```python
from build123d import *

# Parameters (mm, degrees)
F1_DEPTH = 20
F2_R     = 3


with BuildPart() as f1:
    # F0 (on Front) → F1 (new body)
    with BuildSketch(Plane.XZ):
        with BuildLine():
            Line((0, 50), (0, 0))
            Line((0, 0), (200, 0))
            Line((200, 0), (200, 17.131216))
            ThreePointArc((200, 17.131216), (196.384482, 26.898179), (187.280858, 31.956791))
            Line((187.280858, 31.956791), (82.719142, 48.043209))
            ThreePointArc((82.719142, 48.043209), (73.615518, 53.101821), (70, 62.868784))
            Line((70, 62.868784), (70, 137.131216))
            ThreePointArc((70, 137.131216), (73.615518, 146.898179), (82.719142, 151.956791))
            Line((82.719142, 151.956791), (187.280858, 168.043209))
            ThreePointArc((187.280858, 168.043209), (196.384482, 173.101821), (200, 182.868784))
            Line((200, 182.868784), (200, 200))
            Line((200, 200), (0, 200))
            Line((0, 200), (0, 150))
            Line((0, 150), (20, 150))
            Line((20, 150), (20, 50))
            Line((20, 50), (0, 50))
        make_face()
    extrude(amount=F1_DEPTH)

    # F2
    f2_edges = [f1.edges().sort_by_distance(p)[0] for p in [
        (196.384482, -20, 173.101821),
        (200, -20, 191.434392),
        (100, -20, 200),
        (0, -20, 175),
        (10, -20, 150),
        (20, -20, 100),
        (10, -20, 50),
        (0, -20, 25),
        (100, -20, 0),
        (200, -20, 8.565608),
        (196.384482, -20, 26.898179),
        (135, -20, 40),
        (73.615518, -20, 53.101821),
        (70, -20, 100),
        (73.615518, -20, 146.898179),
        (135, -20, 160),
        (196.384482, 0, 173.101821),
        (200, 0, 191.434392),
        (100, 0, 200),
        (0, 0, 175),
        (10, 0, 150),
        (20, 0, 100),
        (10, 0, 50),
        (0, 0, 25),
        (100, 0, 0),
        (200, 0, 8.565608),
        (196.384482, 0, 26.898179),
        (135, 0, 40),
        (73.615518, 0, 53.101821),
        (70, 0, 100),
        (73.615518, 0, 146.898179),
        (135, 0, 160),
    ]]
    fillet(f2_edges, radius=F2_R)


solid = f1.part
```
Check sheet for the modelled part. Datum: model origin and axes. Units: mm. A direction names the side the tool comes from. Round coordinates to 2 decimals unless told otherwise and drop trailing zeros. Order: outer loops, then holes, each group sorted by start corner. A loop starts at its lowest first (then second) coordinate and runs counter-clockwise, first axis right, second up.
1) Section check B-B (z = 74). Record the boundary of the cut face in (x, y), and give its area (3 significant figures).
2) Scan lines: line 1 (Z direction, x = 139.5, y = -4.25); line 2 (Z direction, x = 185.5, y = -16.5); line 3 (X direction, y = -8.75, z = 70.5). Record each from-to range of solid material in increasing order.
3) Mould release check, pull along Z, two halves, no side actions. Record for faces 4 (the cylindrical face through (196.29, -9.9, 172.99)), 5 (the flat face through (200, -10, 8)), 6 (the flat face through (99, -10, 0)), 7 (the cylindrical face through (135.6, -19.1, 160.96)): +Z half, -Z half, draft (parallel to the pull), parting line (faces both ways), or undercut.
4) Section check A-A (y = -10.5). Record the boundary of the cut face in (x, z), and give its area (3 significant figures).
5) Go/stop test with flat-tipped pins: pin 1 Ø8 at (x, y) = (128, -2.5) entering from -Z; pin 2 Ø4 at (y, z) = (-12, 88.5) entering from -X; pin 3 Ø5 at (y, z) = (-3.5, 100.5) entering from +X. Record where each tip stops, or that it passes through.
6) Tool access check on faces 1 (the flat face through (20, -10, 101)), 2 (the cylindrical face through (134.138, -0.902, 39.267)), 3 (the cylindrical face through (73.519, -9.902, 146.785)). Record the directions out of +Z, -Z, +X, -X, +Y, -Y that give a thin tool (end or side, any length) a straight path to the whole face; none if there is none.
Result:
1. outline: (20, -17) arc R3 ccw to (23, -20) - (67, -20) arc R3 ccw to (70, -17) - (70, -3) arc R3 ccw to (67, 0) - (23, 0) arc R3 ccw to (20, -3) - close
1. area: 992 mm2
2. line 1: z = 0 to 39.31, 160.69 to 200
2. line 2: z = 0 to 32.23, 167.77 to 200
2. line 3: x = 20 to 70
3. face 4: undercut
3. face 5: draft
3. face 6: -Z half
3. face 7: undercut
4. outline: (0, 0) - (200, 0) - (200, 17.13) arc R15 ccw to (187.28, 31.96) - (82.72, 48.04) arc R15 cw to (70, 62.87) - (70, 137.13) arc R15 cw to (82.72, 151.96) - (187.28, 168.04) arc R15 ccw to (200, 182.87) - (200, 200) - (0, 200) - (0, 150) - (20, 150) - (20, 50) - (0, 50) - close
4. area: 22,400 mm2
5. pin 1: stops at z = 0
5. pin 2: stops at x = 20
5. pin 3: stops at x = 70
6. face 1: -X, +Y, -Y
6. face 2: +X, +Y
6. face 3: +X, +Y, -Y
